Design review of the part built by this model. Coordinates are the model's own, in mm. Coordinates: 2 decimals unless noted, no trailing zeros. Order: outer loops, then holes, each group sorted by start corner. A loop starts at its lowest first (then second) coordinate and runs counter-clockwise, first axis right, second up. Notation, with made-up numbers: (-17, 21.25) -> (24, 21.25) arc R38 ccw to (24, 60.25) -> close; hole circle Ø1 at (58.5, 23.5). An arc over 180 degrees is marked (long way). Use a Markdown table: item, result. Add a question column.
Q1. Add section B-B (z = 1.5). Count the separate pieces of the cut face and the enclosed holes in it, then the cut area to 3 significant figures.
Q2. Add section A-A (x = 7.5). State the section outline as (y, z) points.
Q3. Add section C-C (y = 87). State the section outline as (x, z) points.
Q4. The part is to be moulded in two halves that separate along X. For faces 1 (the face through (9.127, 99.394, 0.986)), 2 (the face through (-1, 2, 0)), say which applies: pulls with the +X half, pulls with the -X half, needs draft (parallel to the pull), parting line crosses it, or undercut.
Q5. Wall thickness on probe 1 along X at (y, z) = (122, 1.6); probe 2 along X at (y, z) = (77, 1.35); probe 3 along X at (y, z) = (147, 0.6): over which ranges is each line inside the solid? List them lowest first.
from build123d import *

# Parameters (mm, degrees)
SKETCH1_W           = 100
SKETCH1_H           = 300
BOSS_EXTRUDE1_DEPTH = 2
SKETCH2_R           = 1.5
CUT_EXTRUDE1_DEPTH  = 10
SKETCH3_R           = 12.5
CUT_EXTRUDE2_DEPTH  = 10


with BuildPart() as part:
    # Sketch1 → Boss-Extrude1 (new body)
    with BuildSketch(Plane.XY):
        Rectangle(SKETCH1_W, SKETCH1_H)
    extrude(amount=BOSS_EXTRUDE1_DEPTH)

    # Sketch2 → Cut-Extrude1 (cut)
    with BuildSketch(Plane.XY.offset(2)):
        with Locations((-45, 122)):
            Circle(SKETCH2_R)
        with Locations((-45, 77)):
            Circle(SKETCH2_R)
        with Locations((45, 122)):
            Circle(SKETCH2_R)
        with Locations((45, 77)):
            Circle(SKETCH2_R)
        with Locations((-45, 24)):
            Circle(SKETCH2_R)
        with Locations((-45, -21)):
            Circle(SKETCH2_R)
        with Locations((45, 24)):
            Circle(SKETCH2_R)
        with Locations((45, -21)):
            Circle(SKETCH2_R)
        with Locations((-45, -74)):
            Circle(SKETCH2_R)
        with Locations((-45, -119)):
            Circle(SKETCH2_R)
        with Locations((45, -74)):
            Circle(SKETCH2_R)
        with Locations((45, -119)):
            Circle(SKETCH2_R)
        with Locations((16.5, -147)):
            Circle(SKETCH2_R)
        with Locations((-16.5, -147)):
            Circle(SKETCH2_R)
        with Locations((-16.5, -49)):
            Circle(SKETCH2_R)
        with Locations((16.5, -49)):
            Circle(SKETCH2_R)
        with Locations((-16.5, 49)):
            Circle(SKETCH2_R)
        with Locations((16.5, 49)):
            Circle(SKETCH2_R)
        with Locations((-16.5, 147)):
            Circle(SKETCH2_R)
        with Locations((16.5, 147)):
            Circle(SKETCH2_R)
    extrude(amount=-CUT_EXTRUDE1_DEPTH, mode=Mode.SUBTRACT)

    # Sketch3 → Cut-Extrude2 (cut)
    with BuildSketch(Plane(origin=(0, 0, 0), x_dir=(-1, 0, 0), z_dir=(0, 0, -1))):
        with Locations((-7.5, 87)):
            Circle(SKETCH3_R)
    extrude(amount=-CUT_EXTRUDE2_DEPTH, mode=Mode.SUBTRACT)


solid = part.part
Established:
| question | item | result |
|---|---|---|
| 1 | separate pieces | 1 |
| 1 | enclosed holes | 21 |
| 1 | area | 29,400 mm^2 |
| 2 | outline | (-150, 0) -> (74.5, 0) -> (74.5, 2) -> (-150, 2) -> close; (99.5, 0) -> (150, 0) -> (150, 2) -> (99.5, 2) -> close |
| 3 | outline | (-50, 0) -> (-5, 0) -> (-5, 2) -> (-50, 2) -> close; (20, 0) -> (50, 0) -> (50, 2) -> (20, 2) -> close |
| 4 | face 1 | undercut |
| 4 | face 2 | needs draft |
| 5 | probe 1 | -50 to -46.5, -43.5 to 43.5, 46.5 to 50 |
| 5 | probe 2 | -50 to -46.5, -43.5 to 0, 15 to 43.5, 46.5 to 50 |
| 5 | probe 3 | -50 to -18, -15 to 15, 18 to 50 |
